CAD build for the part. Positions are in the model's coordinates, mm. Face numbers are marked on the shaded views. Give positions to 0.01 mm unless a question says otherwise; leave off trailing zeros. Loops run counter-clockwise (first coordinate to the right, second up) from the corner with the lowest first, then second, coordinate; pieces in that order, holes last.
Item 1: Drop flat-ended pins along their axis: P1, Ø3, axis at x = -3.5, y = 1, coming from the -Z side; P2, Ø3, axis at x = 9, y = 5.5, coming from the +Z side; P3, Ø1, axis at y = 3, z = 15.5, coming from the +X side. Give the stop position or say it passes through.
Item 2: Saw through at D-D on x = -8. Give the cut face in (y, z), plus the area to 3 significant figures.
Item 3: Saw through at B-B on y = 5.25. Give the cut face in (x, z), plus the area to 3 significant figures.
Item 4: Mould opens along Z. For the marked faces 1, 2 and 3 say: released by +Z, released by -Z, zero draft, split by the parting line, or undercut.
Item 5: Probe probe 1 along Z at (x, y) = (0, 7.5); probe 2 along X at (y, z) = (6, 16); probe 3 along Z at (x, y) = (11, 3). List the from-to ranges inside material, lowest first.
Item 6: Saw through at A-A on x = 0. Give the cut face in (y, z).
Item 7: Saw through at C-C on z = 0. Give the cut face in (x, y), plus the area to 3 significant figures.
Autodesk Inventor part; units mm, degrees
ref_plane "YZ Plane" through (0, 0, 0) normal (1, 0, 0) x (0, 1, 0)
ref_plane "XZ Plane" through (0, 0, 0) normal (0, 1, 0) x (-1, 0, 0)
ref_plane "XY Plane" through (0, 0, 0) normal (0, 0, 1) x (1, 0, 0)
sketch "Sketch1" plane through (0, 0, 0) normal (0, 1, 0) x (-1, 0, 0)
  circle A0 centre (0, 0) radius 25
  dimension "d0" = 50
extrude "Extrusion1" add sketch "Sketch1" along normal blind 10
sketch "Sketch2" plane through (0, 10, 0) normal (0, 1, 0) x (1, 0, 0)
  arc A0 (-2.1, -3.2863) -> (-2.1, 3.2863) centre (0, 0) ccw
  line L0 (-2.1, -3.2863) -> (-2.1, 3.2863)
  dimension "d3" = 7.8
  dimension "d4" = 2.1
extrude "Extrusion2" cut sketch "Sketch2" against normal up to surface (10 mm away)
sketch "Sketch3" plane through (0, 10, 0) normal (0, 1, 0) x (1, 0, 0)
  line L0 (-2.1, -3.2863) -> (-2.1, 3.2863)
  arc A0 (-2.1, -3.2863) -> (-2.1, 3.2863) centre (0, 0) ccw
  circle A1 centre (0, 0) radius 25
  line L1 (-23.5896, -0.7) -> (-5.2536, -0.7)
  line L2 (-23.5896, 0.7) -> (-5.2536, 0.7)
  line L3 (11.1886, 20.7792) -> (2.0206, 4.8997)
  line L4 (12.401, 20.0792) -> (3.233, 4.1997)
  line L5 (12.401, -20.0792) -> (3.233, -4.1997)
  line L6 (11.1886, -20.7792) -> (2.0206, -4.8997)
  arc A2 (3.233, -4.1997) -> (3.233, 4.1997) centre (0, 0) ccw
  arc A3 (12.401, -20.0792) -> (12.401, 20.0792) centre (0, 0) ccw
  arc A4 (2.0206, 4.8997) -> (-5.2536, 0.7) centre (0, 0) ccw
  arc A5 (-5.2536, -0.7) -> (2.0206, -4.8997) centre (0, 0) ccw
  arc A6 (11.1886, 20.7792) -> (-23.5896, 0.7) centre (0, 0) ccw
  arc A7 (-23.5896, -0.7) -> (11.1886, -20.7792) centre (0, 0) ccw
  dimension "d9" = 1.4
  dimension "d12" = 360
extrude "Extrusion3" cut sketch "Sketch3" against normal through all contours L1 A5 L6 A7 | A6 L3 A4 L2 | A3 L5 A2 L4
properties part number "Wheel"
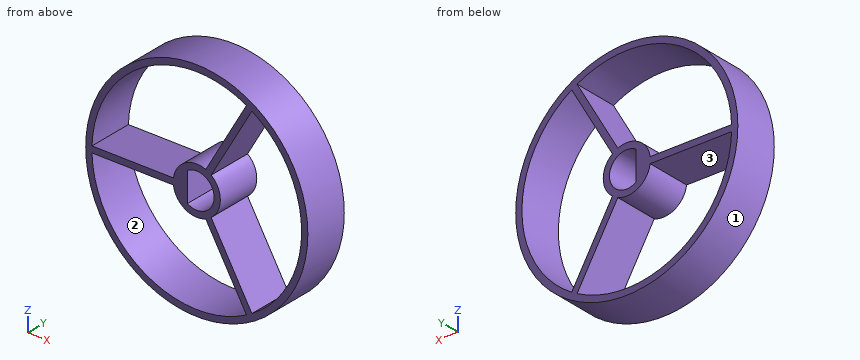
Results below:
1. P1: stops at z = -24.92
1. P2: stops at z = 23.85
1. P3: stops at x = 20
2. outline: (0, -23.69) - (10, -23.69) - (10, -22.2) - (0, -22.2) - close; (0, -0.7) - (10, -0.7) - (10, 0.7) - (0, 0.7) - close; (0, 22.2) - (10, 22.2) - (10, 23.69) - (0, 23.69) - close
2. area: 43.7 mm2
3. outline: circle Ø50 at (0, 0); hole (-23.59, -0.7) arc R23.6 ccw to (11.19, -20.78) - (2.02, -4.9) arc R5.3 cw to (-5.25, -0.7) - close; hole (-23.59, 0.7) - (-5.25, 0.7) arc R5.3 cw to (2.02, 4.9) - (11.19, 20.78) arc R23.6 ccw to start; hole (-2.1, -3.29) arc R3.9 ccw (long way) to (-2.1, 3.29) - close; hole (3.23, -4.2) - (12.4, -20.08) arc R23.6 ccw to (12.4, 20.08) - (3.23, 4.2) arc R5.3 cw to start
3. area: 339 mm2
4. face 1: split by the parting line
4. face 2: undercut
4. face 3: undercut
5. probe 1: z = -25 to -23.6, -5.3 to -3.9, 3.9 to 5.3, 23.6 to 25
5. probe 2: x = -19.21 to -17.35, 8.43 to 10.05, 17.35 to 19.21
5. probe 3: z = -22.45 to -20.88, -20.45 to -17.65, 17.65 to 20.45, 20.88 to 22.45
6. outline: (0, -25) - (10, -25) - (10, -23.6) - (0, -23.6) - close; (0, -5.3) - (10, -5.3) - (10, -3.9) - (0, -3.9) - close; (0, 3.9) - (10, 3.9) - (10, 5.3) - (0, 5.3) - close; (0, 23.6) - (10, 23.6) - (10, 25) - (0, 25) - close
7. outline: (-25, 0) - (-2.1, 0) - (-2.1, 10) - (-25, 10) - close; (3.9, 0) - (5.3, 0) - (5.3, 10) - (3.9, 10) - close; (23.6, 0) - (25, 0) - (25, 10) - (23.6, 10) - close
7. area: 257 mm2
